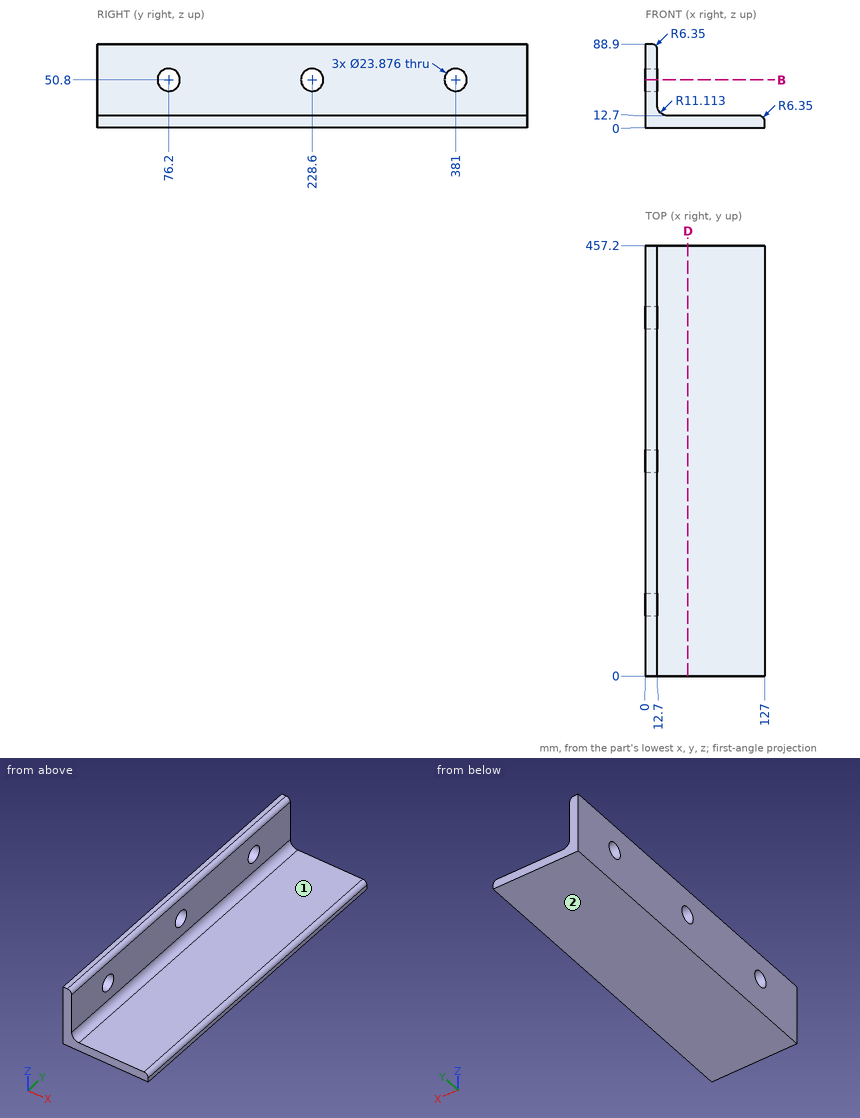
The figure shows three views and two pictorial views of one solid part (mm, origin at its lowest corner). Answer the questions. A direction names the side the tool comes from. Coordinates: 2 decimals unless noted, no trailing zeros. Order: outer loops, then holes, each group sorted by start corner. A loop starts at its lowest first (then second) coordinate and runs counter-clockwise, first axis right, second up.
Q1. A cutting plane is placed at D-D, the plane x = 45. Write down the section's boundary in (y, z).
Q2. Consider line 1 (Y direction, x = 4, z = 50); line 2 (Z direction, x = 4, y = 228.6); line 3 (X direction, y = 55, z = 79). Determine where each line is inside the solid, lowest interval first.
Q3. A cutting plane is placed at B-B, the plane z = 50.8. Write down the section's boundary in (x, y), and give its area (3 significant figures).
Q4. Given P1, Ø2, axis at x = 38.5, y = 292, coming from the +Z side; P2, Ø2, axis at y = 207.5, z = 60, coming from the +X side; P3, Ø8, axis at y = 371, z = 53.5, coming from the -X side; P4, Ø2, axis at y = 239, z = 14.5, coming from the +X side (1 decimal), each flat-ended and moving along its own axis, determine where each tip first touches the part or whether it passes through.
Q5. Which of the six approach directions +Z, -Z, +X, -X, +Y, -Y give full straight-line access (tool end or side, diameter ignored) to the marked faces 1 and 2?
Answers follow:
1. outline: (0, 0) - (457.2, 0) - (457.2, 12.7) - (0, 12.7) - close
2. line 1: y = 0 to 64.29, 88.11 to 216.69, 240.51 to 369.09, 392.91 to 457.2
2. line 2: z = 0 to 38.86, 62.74 to 88.9
2. line 3: x = 0 to 12.7
3. outline: (0, 0) - (12.7, 0) - (12.7, 64.26) - (0, 64.26) - close; (0, 88.14) - (12.7, 88.14) - (12.7, 216.66) - (0, 216.66) - close; (0, 240.54) - (12.7, 240.54) - (12.7, 369.06) - (0, 369.06) - close; (0, 392.94) - (12.7, 392.94) - (12.7, 457.2) - (0, 457.2) - close
3. area: 4,900 mm2
4. P1: stops at z = 12.7
4. P2: stops at x = 12.7
4. P3: stops at x = 0
4. P4: stops at x = 19.7
5. face 1: +Z, +X, +Y, -Y
5. face 2: -Z, +X, -X, +Y, -Y
